Source: CAD feature listing. Evaluate the final solid. Frame: model axes, mm. A direction names the side the tool comes from. Coordinates: 2 decimals unless noted, no trailing zeros. Loops run counter-clockwise (first coordinate to the right, second up) from the corner with the lowest first, then second, coordinate; pieces in that order, holes last.
```python
from build123d import *

# Parameters (mm, degrees)
SKETCH_1_R          = 1.45
SKETCH_1_W          = 30
SKETCH_1_H          = 13
EXTRUDE_1_DEPTH     = 3
SKETCH_2_W          = 80
SKETCH_2_H          = 2
CUT_EXTRUDE_1_DEPTH = 59.005258382
FILLET_1_R          = 3


with BuildPart() as part:
    # 草图1 → 凸台-拉伸1 (new body)
    with BuildSketch(Plane(origin=(0, 0, 0), x_dir=(1, 0, 0), z_dir=(0, 1, 0))):
        Polygon((-20, -7.6), (-20, 7.6), (-40, 7.6), (-40, 41.9), (40, 41.9), (40, 7.6), (20, 7.6), (20, -7.6), (20.435801373, -13.585557258), (22.396449617, -40.514275357), (7.436050673, -41.603524381), (5.475402429, -14.674806282), (-20, -16.529640324), align=None)
        with Locations(Location((-35, 13.4, 0), (0, 0, 270))):
            Circle(SKETCH_1_R, mode=Mode.SUBTRACT)
        with Locations(Location((-35, 36.4, 0), (0, 0, 270))):
            Circle(SKETCH_1_R, mode=Mode.SUBTRACT)
        with Locations(Location((35, 13.4, 0), (0, 0, 90))):
            Circle(SKETCH_1_R, mode=Mode.SUBTRACT)
        with Locations(Location((35, 36.4, 0), (0, 0, 90))):
            Circle(SKETCH_1_R, mode=Mode.SUBTRACT)
        with Locations(Location((-14.029429392, -8.57507717, 0), (0, 0, 270))):
            Circle(SKETCH_1_R, mode=Mode.SUBTRACT)
        with Locations(Location((10.904568848, -6.759662129, 0), (0, 0, 270))):
            Circle(SKETCH_1_R, mode=Mode.SUBTRACT)
        with Locations(Location((13.827001121, -26.098500925, 0), (0, 0, 270))):
            Circle(SKETCH_1_R, mode=Mode.SUBTRACT)
        with Locations(Location((14.407933934, -34.077380362, 0), (0, 0, 270))):
            Circle(SKETCH_1_R, mode=Mode.SUBTRACT)
        with Locations((-20, 24.75)):
            Rectangle(SKETCH_1_W, SKETCH_1_H, mode=Mode.SUBTRACT)
        with Locations((20, 24.75)):
            Rectangle(SKETCH_1_W, SKETCH_1_H, mode=Mode.SUBTRACT)
    extrude(amount=EXTRUDE_1_DEPTH)

    # 草图2 → 切除-拉伸1 (cut, through all)
    with BuildSketch(Plane(origin=(0, 3, 0), x_dir=(1, 0, 0), z_dir=(0, 1, 0))):
        with Locations((0, 40.9)):
            Rectangle(SKETCH_2_W, SKETCH_2_H)
    extrude(amount=-CUT_EXTRUDE_1_DEPTH, mode=Mode.SUBTRACT)

    # 圆角1
    # the kernel refuses this fillet: 3 mm, written as the material it adds along each edge
    with BuildSketch(Plane(origin=(20, 0, -7.6), x_dir=(0, 0, 1), z_dir=(0, 1, 0)), Plane(origin=(5.475402429, 0, 14.674806282), x_dir=(-0.9973599295981227, 0, 0.07261660162819321), z_dir=(0, 1, 0)), Plane(origin=(-35, 0, -31.25), x_dir=(0, 0, 1), z_dir=(0, 1, 0)), Plane(origin=(-35, 0, -18.25), x_dir=(1, 0, 0), z_dir=(0, 1, 0)), Plane(origin=(5, 0, -18.25), x_dir=(1, 0, 0), z_dir=(0, 1, 0)), Plane(origin=(5, 0, -31.25), x_dir=(0, 0, 1), z_dir=(0, 1, 0))) as fillet_1_piece_1:
        with BuildLine():
            CenterArc((FILLET_1_R, FILLET_1_R), FILLET_1_R, 180, 90)
            Line((0, FILLET_1_R), (0, 0))
            Line((0, 0), (FILLET_1_R, 0))
        make_face()
    extrude(amount=3)
    with BuildSketch(Plane(origin=(20, 0, 7.6), x_dir=(0.07261660162820198, 0, 0.9973599295981221), z_dir=(0, 1, 0))) as fillet_1_piece_2:
        with BuildLine():
            CenterArc((FILLET_1_R * 0.0363562923998, FILLET_1_R), FILLET_1_R, 265.835709886, 4.164290114)
            Line((-FILLET_1_R * 0.0362603092284, FILLET_1_R * 0.00264007040188), (0, 0))
            Line((0, 0), (FILLET_1_R * 0.0363562923998, 0))
        make_face()
    extrude(amount=3)
    with BuildSketch(Plane(origin=(-20, 0, -7.6), x_dir=(0, 0, 1), z_dir=(0, 1, 0)), Plane(origin=(-5, 0, -18.25), x_dir=(-1, 0, 0), z_dir=(0, 1, 0)), Plane(origin=(-5, 0, -31.25), x_dir=(0, 0, 1), z_dir=(0, 1, 0)), Plane(origin=(35, 0, -18.25), x_dir=(-1, 0, 0), z_dir=(0, 1, 0)), Plane(origin=(35, 0, -31.25), x_dir=(0, 0, 1), z_dir=(0, 1, 0))) as fillet_1_piece_3:
        with BuildLine():
            CenterArc((FILLET_1_R, -FILLET_1_R), FILLET_1_R, 90, 90)
            Line((0, -FILLET_1_R), (0, 0))
            Line((0, 0), (FILLET_1_R, 0))
        make_face()
    extrude(amount=3)
    # the kernel refuses this fillet: 3 mm, written as the material it takes off along each edge
    with BuildSketch(Plane(origin=(-40, 10.5, -39.9), x_dir=(1, 0, 0), z_dir=(0, -1, 0)), Plane(origin=(40, 10.5, -39.9), x_dir=(0, 0, 1), z_dir=(0, -1, 0)), Plane(origin=(-40, -7.5, -7.6), x_dir=(1, 0, 0), z_dir=(0, 1, 0))) as fillet_1_2_piece_1:
        with BuildLine():
            CenterArc((FILLET_1_R, FILLET_1_R), FILLET_1_R, 180, 90)
            Line((0, FILLET_1_R), (0, 0))
            Line((0, 0), (FILLET_1_R, 0))
        make_face()
    extrude(amount=18, mode=Mode.SUBTRACT)
    with BuildSketch(Plane(origin=(22.396449617, -7.5, 40.514275357), x_dir=(-0.9973599295981227, 0, 0.07261660162819322), z_dir=(0, 1, 0)), Plane(origin=(7.436050673, -7.5, 41.603524381), x_dir=(-0.07261660162819356, 0, -0.9973599295981227), z_dir=(0, 1, 0)), Plane(origin=(40, -7.5, -7.6), x_dir=(-1, 0, 0), z_dir=(0, 1, 0))) as fillet_1_2_piece_2:
        with BuildLine():
            CenterArc((FILLET_1_R, -FILLET_1_R), FILLET_1_R, 90, 90)
            Line((0, -FILLET_1_R), (0, 0))
            Line((0, 0), (FILLET_1_R, 0))
        make_face()
    extrude(amount=18, mode=Mode.SUBTRACT)
    with BuildSketch(Plane(origin=(-20, -8.065919107, 16.529640324), x_dir=(0, 0, -1), z_dir=(0, 1, 0))) as fillet_1_2_piece_3:
        with BuildLine():
            CenterArc((FILLET_1_R * 1.07545588087, -FILLET_1_R), FILLET_1_R, 90, 94.164290114)
            Line((FILLET_1_R * 0.0780959512697, -FILLET_1_R * 1.07261660163), (0, 0))
            Line((0, 0), (FILLET_1_R * 1.07545588087, 0))
        make_face()
    extrude(amount=19.131838213, mode=Mode.SUBTRACT)


solid = part.part
```
Q1. Reachability of faces 1 (the flat face through (-7.015, 1.479, 15.584)), 2 (the flat face through (-30, 1, -7.6)), 3 (the flat face through (20, 1, -31.25)) from +Z, -Z, +X, -X, +Y, -Y: full face, straight path, thin tool, end or side. Return the list, or none.
Q2. First-contact query: pin 1 Ø2.5 at (x, z) = (-14.03, 8.58) entering from -Y; pin 2 Ø0.9 at (x, y) = (21, 1) entering from +Z. Flat tips, straight axial feed; report the tip coordinate or a pass-through.
Q3. Material intervals for line 1 along Z through (x, y) = (11.5, 0.5); line 2 along Z through (x, y) = (23.5, 1.2); line 3 along Z through (x, y) = (12.5, 2.95), sorted ascending.
Q4. Section query C-C on y = 2.4. Count the separate pieces of the cut face and the enclosed holes in it, then the cut area to 3 significant figures.
Q5. Section query A-A on x = 31. Return the cut outline in (y, z).
Q6. Draft query along X for faces 4 (the flat face through (-1, 2, -39.9)), 5 (the flat face through (14.979, 1.479, 41.054)), 6 (the flat face through (-40, 1, -24)), 7 (the cylindrical face through (-5.9, 1.48, -19.11)). Return one class per face: released by +X, released by -X, zero draft, split by the parting line, or undercut.
Q7. Section query B-B on z = -26. Return the cut outline in (x, y), then the cut area to 3 significant figures.
Q8. Section query D-D on x = -3. Return the cut outline in (y, z), then the cut area to 3 significant figures.
Resolved:
1. face 1: +Z, +Y, -Y
1. face 2: +Z, -X, +Y, -Y
1. face 3: +Y, -Y
2. pin 1: passes through
2. pin 2: stops at z = 40.41
3. line 1: z = -39.9 to -31.25, -18.25 to 5.44, 8.08 to 41.31
3. line 2: z = -39.9 to -31.25, -18.25 to -7.6
3. line 3: z = -39.9 to -31.25, -18.25 to 25.51, 26.68 to 41.23
4. separate pieces: 1
4. enclosed holes: 10
4. area: 3,070 mm2
5. outline: (0, -39.9) - (3, -39.9) - (3, -31.25) - (0, -31.25) - close; (0, -18.25) - (3, -18.25) - (3, -7.6) - (0, -7.6) - close
6. face 4: zero draft
6. face 5: released by +X
6. face 6: released by -X
6. face 7: undercut
7. outline: (-40, 0) - (-35, 0) - (-35, 3) - (-40, 3) - close; (-5, 0) - (5, 0) - (5, 3) - (-5, 3) - close; (35, 0) - (40, 0) - (40, 3) - (35, 3) - close
7. area: 60.0 mm2
8. outline: (0, -39.9) - (3, -39.9) - (3, 15.29) - (0, 15.29) - close
8. area: 166 mm2
